Geometry: final body of the model. Coordinates: model frame, mm. Face numbers are marked on the shaded views. A direction names the side the tool comes from. Give positions to 0.01 mm unless a question says otherwise; leave off trailing zeros. Loops run counter-clockwise (first coordinate to the right, second up) from the corner with the lowest first, then second, coordinate; pieces in that order, holes last.
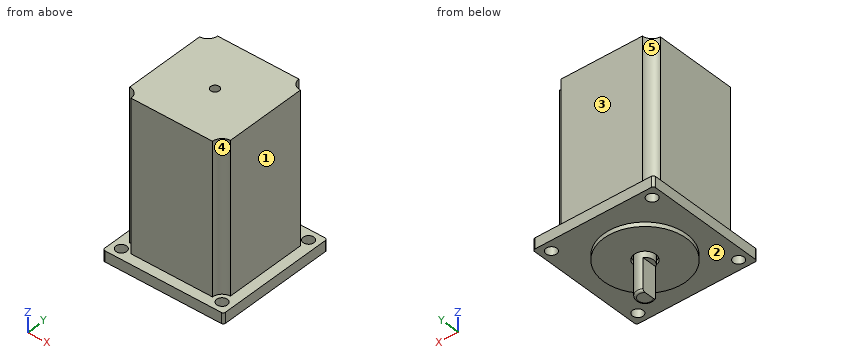
from build123d import *

# Parameters (mm, degrees)
SKETCH_W      = 56.4
SKETCH_H      = 56.4
SKETCH_R      = 2.5
SKETCH_R_2    = 2
PAD_DEPTH     = 5
SKETCH001_R   = 2
PAD001_DEPTH  = 70
SKETCH002_R   = 19.2
SKETCH002_R_2 = 5
PAD002_DEPTH  = 2
SKETCH005_R   = 4
PAD003_DEPTH  = 19
POCKET_DEPTH  = 15
FILLET_R      = 1
FILLET001_R   = 1


with BuildPart() as part:
    # Sketch → Pad (new body)
    with BuildSketch(Plane.XY):
        Rectangle(SKETCH_W, SKETCH_H)
        with Locations((-23.5, 23.5)):
            Circle(SKETCH_R, mode=Mode.SUBTRACT)
        with Locations((23.5, 23.5)):
            Circle(SKETCH_R, mode=Mode.SUBTRACT)
        with Locations((-23.5, -23.5)):
            Circle(SKETCH_R, mode=Mode.SUBTRACT)
        with Locations((23.5, -23.5)):
            Circle(SKETCH_R, mode=Mode.SUBTRACT)
        Circle(SKETCH_R_2, mode=Mode.SUBTRACT)
    extrude(amount=PAD_DEPTH)

    # Sketch001 (on Face11 of Pad) → Pad001 (join)
    with BuildSketch(Plane.XY.offset(5)):
        with BuildLine():
            ThreePointArc((-19, -23.5), (-20.318019, -20.318019), (-23.5, -19))
            Line((-23.5, -19), (-23.5, 19))
            ThreePointArc((-23.5, 19), (-20.318019, 20.318019), (-19, 23.5))
            Line((-19, 23.5), (19, 23.5))
            ThreePointArc((19, 23.5), (20.318019, 20.318019), (23.5, 19))
            Line((23.5, -19), (23.5, 19))
            ThreePointArc((23.5, -19), (20.318019, -20.318019), (19, -23.5))
            Line((19, -23.5), (-19, -23.5))
        make_face()
        Circle(SKETCH001_R, mode=Mode.SUBTRACT)
    extrude(amount=PAD001_DEPTH)

    # Sketch002 (on Face4 of Pad001) → Pad002 (join)
    with BuildSketch(Plane(origin=(0, 0, 0), x_dir=(1, 0, 0), z_dir=(0, 0, -1))):
        Circle(SKETCH002_R)
        Circle(SKETCH002_R_2, mode=Mode.SUBTRACT)
    extrude(amount=PAD002_DEPTH)

    # Sketch005 (on Face24 of Pad002) → Pad003 (join)
    with BuildSketch(Plane(origin=(0, 0, 0), x_dir=(1, 0, 0), z_dir=(0, 0, -1))):
        Circle(SKETCH005_R)
    extrude(amount=PAD003_DEPTH)

    # Sketch004 → Pocket (cut)
    with BuildSketch(Plane(origin=(0, 0, -19), x_dir=(1, 0, 0), z_dir=(0, 0, -1))):
        with BuildLine():
            ThreePointArc((-2, 3.464102), (-4, 0), (-2, -3.464102))
            Line((-2, 3.464102), (-2, -3.464102))
        make_face()
    extrude(amount=-POCKET_DEPTH, mode=Mode.SUBTRACT)

    # Fillet
    fillet_edges = [part.edges().sort_by_distance(p)[0] for p in [
        (-28.2, 28.2, 2.5),
        (-28.2, -28.2, 2.5),
        (28.2, 28.2, 2.5),
        (28.2, -28.2, 2.5),
    ]]
    fillet(fillet_edges, radius=FILLET_R)

    # Fillet001
    fillet001_edges = [part.edges().sort_by_distance(p)[0] for p in [
        (2, 3.464102, -19),
    ]]
    fillet(fillet001_edges, radius=FILLET001_R)


solid = part.part
Item 1: Set-up query: the marked faces 1, 2, 3, 4 and 5. Return all of +Z, -Z, +X, -X, +Y, -Y with unobstructed straight access to the full face (end or side cutting, diameter ignored); none if empty.
Values follow:
face 1: +Z, +X, +Y, -Y
face 2: -Z
face 3: +Z, +X, -X, +Y
face 4: +Z, +X, -Y
face 5: +Z, -X, +Y
Item 2: Section query C-C on x = -22. Return loops of the section in (y, z).
Values follow:
outline: (-28.2, 0) - (-25.5, 0) - (-25.5, 5) - (-28.2, 5) - close; (-21.5, 0) - (21.5, 0) - (21.5, 5) - (19.26, 5) - (19.26, 75) - (-19.26, 75) - (-19.26, 5) - (-21.5, 5) - close; (25.5, 0) - (28.2, 0) - (28.2, 5) - (25.5, 5) - close
Item 3: Ray query, probe 1 along Y at (x, z) = (-23.5, 2.1); probe 2 along X at (y, z) = (-23, 3). Return the intervals inside material, ascending.
Values follow:
probe 1: y = -28.2 to -26, -21 to 21, 26 to 28.2
probe 2: x = -28.2 to -25.95, -21.05 to 21.05, 25.95 to 28.2
Item 4: Section query D-D on y = 0. Return loops of the section in (x, z).
Values follow:
outline: (-28.2, 0) - (-19.2, 0) - (-19.2, -2) - (-5, -2) - (-5, 0) - (-4, 0) - (-4, -4) - (-2, -4) - (-2, -19) - (3, -19) arc R1 ccw to (4, -18) - (4, 0) - (5, 0) - (5, -2) - (19.2, -2) - (19.2, 0) - (28.2, 0) - (28.2, 5) - (23.5, 5) - (23.5, 75) - (2, 75) - (2, 0) - (-2, 0) - (-2, 75) - (-23.5, 75) - (-23.5, 5) - (-28.2, 5) - close
Item 5: Section query A-A on z = 67. Return loops of the section in (x, y).
Values follow:
outline: (-23.5, -19) arc R4.5 cw to (-19, -23.5) - (19, -23.5) arc R4.5 cw to (23.5, -19) - (23.5, 19) arc R4.5 cw to (19, 23.5) - (-19, 23.5) arc R4.5 cw to (-23.5, 19) - close; hole circle Ø4 at (0, 0)
Item 6: Section query B-B on y = 24.5. Return loops of the section in (x, z), plus the area to 3 significant figures.
Values follow:
outline: (-28.2, 0) - (-25.79, 0) - (-25.79, 5) - (-28.2, 5) - close; (-21.21, 0) - (21.21, 0) - (21.21, 5) - (-21.21, 5) - close; (25.79, 0) - (28.2, 0) - (28.2, 5) - (25.79, 5) - close
area: 236 mm2
Item 7: Pin query (flat end, axial travel): pin 1 (1.5 mm diameter, centred on x = -15, z = 62.5, fed in from +Y); pin 2 (1 mm diameter, centred on y = -12, z = 61.5, fed in from +X); pin 3 (5.5 mm diameter, centred on y = -1.5, z = -14, fed in from -X). Return the tip coordinate at first contact, or that it passes through.
Values follow:
pin 1: stops at y = 23.5
pin 2: stops at x = 23.5
pin 3: stops at x = -2
